Source: CAD feature listing. Evaluate the final solid. Frame: model axes, mm. A direction names the side the tool comes from. Give positions to 0.01 mm unless a question says otherwise; leave off trailing zeros. Loops run counter-clockwise (first coordinate to the right, second up) from the corner with the lowest first, then second, coordinate; pieces in that order, holes last. Notation, with made-up numbers: M 75.25,4 L 89.25,4 A33 cw 89.25,43 Z; hole C 57,5.25 d11. An arc over 180 degrees is marked long. Write item = value, one per line.
from build123d import *

# Parameters (mm, degrees)
BOSS_EXTRUDE1_DEPTH = 38.1
SKETCH2_R           = 19.05
BOSS_EXTRUDE2_DEPTH = 203.2
SKETCH4_W           = 254
SKETCH4_H           = 38.1
BOSS_EXTRUDE3_DEPTH = 177.8
CUT_EXTRUDE3_DEPTH  = 38.1
SKETCH8_R           = 6.35
CUT_EXTRUDE4_DEPTH  = 432.286091243
BOSS_EXTRUDE4_REACH = 409.638
SKETCH9_W           = 50.8
SKETCH9_H           = 38.1
BOSS_EXTRUDE5_DEPTH = 50.8
SKETCH13_W          = 63.5
SKETCH13_H          = 38.1
BOSS_EXTRUDE6_DEPTH = 50.8
CUT_EXTRUDE7_DEPTH  = 438.78172929
FILLET1_R           = 2.54
SKETCH12_R          = 9.525
CUT_EXTRUDE5_DEPTH  = 438.78172929


with BuildPart() as part:
    # Sketch1 → Boss-Extrude1 (new body)
    with BuildSketch(Plane.XY):
        with BuildLine():
            Line((228.6, 38.1), (-228.6, 38.1))
            ThreePointArc((-228.6, 38.1), (-247.65, 19.05), (-228.6, 0))
            Line((-228.6, 0), (228.6, 0))
            ThreePointArc((228.6, 0), (247.65, 19.05), (228.6, 38.1))
        make_face()
    boss_extrude1 = extrude(amount=BOSS_EXTRUDE1_DEPTH)

    # Sketch2 → Boss-Extrude2 (add)
    with BuildSketch(Plane.XY.offset(38.1)):
        with Locations(Location((-228.6, 19.05, 0), (0, 0, 270))):
            Circle(SKETCH2_R)
        with Locations(Location((228.6, 19.05, 0), (0, 0, 90))):
            Circle(SKETCH2_R)
    boss_extrude2 = extrude(amount=BOSS_EXTRUDE2_DEPTH)

    # Mirror3: Boss-Extrude1, Boss-Extrude2 across plane
    add(boss_extrude1.mirror(Plane.XY.offset(139.7)))
    add(boss_extrude2.mirror(Plane.XY.offset(139.7)))

    # Sketch4 → Boss-Extrude3 (add)
    with BuildSketch(Plane(origin=(0, 38.1, 0), x_dir=(1, 0, 0), z_dir=(0, 1, 0))):
        with Locations((-101.6, -260.35)):
            Rectangle(SKETCH4_W, SKETCH4_H)
    boss_extrude3 = extrude(amount=BOSS_EXTRUDE3_DEPTH)

    # Sketch7 → Cut-Extrude3 (cut)
    with BuildSketch(Plane.XY.offset(279.4)):
        Polygon((-228.6, 38.1), (-127, 215.9), (-228.6, 215.9), align=None)
        Polygon((-76.2, 215.9), (25.4, 38.1), (25.4, 215.9), align=None)
        Polygon((-127, 164.704663298), (-199.345521885, 38.1), (-127, 38.1), align=None)
        Polygon((-76.2, 164.704663298), (-76.2, 38.1), (-3.854478115, 38.1), align=None)
    cut_extrude3 = extrude(amount=-CUT_EXTRUDE3_DEPTH, mode=Mode.SUBTRACT)

    # Mirror4: Boss-Extrude3, Cut-Extrude3 across plane
    add(boss_extrude3.mirror(Plane.XY.offset(139.7)))
    add(cut_extrude3.mirror(Plane.XY.offset(139.7)), mode=Mode.SUBTRACT)

    # Sketch8 → Cut-Extrude4 (cut, through all)
    with BuildSketch(Plane.XY.offset(279.4)):
        with Locations((-228.6, 19.05)):
            Circle(SKETCH8_R)
        with Locations((127, 19.05)):
            Circle(SKETCH8_R)
    extrude(amount=-CUT_EXTRUDE4_DEPTH, mode=Mode.SUBTRACT)

    # Sketch9 → Boss-Extrude4 (add, up to next)
    with BuildSketch(Plane(origin=(0, 0, 241.3), x_dir=(-1, 0, 0), z_dir=(0, 0, -1)), mode=Mode.PRIVATE) as boss_extrude4_sk1:
        with Locations((101.6, 196.85)):
            Rectangle(SKETCH9_W, SKETCH9_H)
    boss_extrude4_tool1 = extrude(boss_extrude4_sk1.sketch, amount=BOSS_EXTRUDE4_REACH, mode=Mode.PRIVATE) - part.part
    add(boss_extrude4_tool1.solids().sort_by_distance((-101.6, 196.85, 241.3))[0])

    # Sketch10 → Boss-Extrude5 (add)
    with BuildSketch(Plane.XZ.offset(-177.8)):
        with BuildLine():
            Line((-76.2, 177.8), (-38.1, 177.8))
            Line((-38.1, 177.8), (-38.1, 164.293444248))
            ThreePointArc((-38.1, 164.293444248), (-57.15, 139.7), (-38.1, 115.106555752))
            Line((-38.1, 115.106555752), (-38.1, 101.6))
            Line((-38.1, 101.6), (-76.2, 101.6))
            Line((-76.2, 101.6), (-76.2, 177.8))
        make_face()
    extrude(amount=-BOSS_EXTRUDE5_DEPTH)

    # Sketch13 → Boss-Extrude6 (add)
    with BuildSketch(Plane(origin=(0, 38.1, 0), x_dir=(1, 0, 0), z_dir=(0, 1, 0))):
        with Locations((196.85, -260.35)):
            Rectangle(SKETCH13_W, SKETCH13_H)
        with Locations((196.85, -19.05)):
            Rectangle(SKETCH13_W, SKETCH13_H)
    extrude(amount=BOSS_EXTRUDE6_DEPTH)

    # Sketch14 → Cut-Extrude7 (cut, through all)
    with BuildSketch(Plane(origin=(0, 0, 0), x_dir=(-1, 0, 0), z_dir=(0, 0, -1))):
        Polygon((-177.8, 88.9), (-165.1, 38.1), (-165.1, 88.9), align=None)
        Polygon((-228.6, 38.1), (-215.9, 88.9), (-228.6, 88.9), align=None)
    extrude(amount=-CUT_EXTRUDE7_DEPTH, mode=Mode.SUBTRACT)

    # Fillet1
    # the kernel refuses this fillet: 2.54 mm, written as the material it adds along each edge
    with BuildSketch(Plane(origin=(25.4, 38.1, 38.1), x_dir=(1, 0, 0), z_dir=(0, 0, -1))) as fillet1_piece_1:
        with BuildLine():
            CenterArc((FILLET1_R * 0.580322535471, -FILLET1_R), FILLET1_R, 90, 60.255118703)
            Line((-FILLET1_R * 0.287920606653, -FILLET1_R * 0.503861061643), (0, 0))
            Line((0, 0), (FILLET1_R * 0.580322535471, 0))
        make_face()
    extrude(amount=38.1)
    with BuildSketch(Plane(origin=(-76.2, 215.9, 177.8), x_dir=(-1, 0, 0), z_dir=(0, 0, -1))) as fillet1_piece_2:
        with BuildLine():
            CenterArc((FILLET1_R, FILLET1_R), FILLET1_R, 180, 90)
            Line((0, FILLET1_R), (0, 0))
            Line((0, 0), (FILLET1_R, 0))
        make_face()
    extrude(amount=76.2)
    with BuildSketch(Plane(origin=(165.1, 38.1, 241.3), x_dir=(-1, 0, 0), z_dir=(0, 0, 1))) as fillet1_piece_3:
        with BuildLine():
            CenterArc((FILLET1_R * 0.780776406404, -FILLET1_R), FILLET1_R, 90, 75.963756532)
            Line((-FILLET1_R * 0.189366093741, -FILLET1_R * 0.757464374964), (0, 0))
            Line((0, 0), (FILLET1_R * 0.780776406404, 0))
        make_face()
    extrude(amount=38.1)
    with BuildSketch(Plane(origin=(165.1, 38.1, 38.1), x_dir=(-1, 0, 0), z_dir=(0, 0, -1))) as fillet1_piece_4:
        with BuildLine():
            CenterArc((FILLET1_R * 0.780776406404, FILLET1_R), FILLET1_R, 194.036243468, 75.963756532)
            Line((-FILLET1_R * 0.189366093741, FILLET1_R * 0.757464374964), (0, 0))
            Line((0, 0), (FILLET1_R * 0.780776406404, 0))
        make_face()
    extrude(amount=38.1)
    with BuildSketch(Plane(origin=(-228.6, 38.1, 279.4), x_dir=(-0.9993924886813553, -0.03485188039815198, 0), z_dir=(0, 0, -1))) as fillet1_piece_5:
        with BuildLine():
            CenterArc((1.416380419, 2.538456921), FILLET1_R, 211.742151423, 56.260578451)
            Line((-0.743697302, 1.202169438), (0, 0))
            ThreePointArc((0, 0), (0.663928322, 0.011573091), (1.327856643, 0))
        make_face()
    extrude(amount=38.1)
    with BuildSketch(Plane(origin=(228.6, 38.1, 279.4), x_dir=(0.9989173866825803, -0.04651940007399378, 0), z_dir=(0, 0, -1))) as fillet1_piece_6:
        with BuildLine():
            CenterArc((1.890548419, -2.537250162), FILLET1_R, 92.66632756, 70.631101413)
            Line((-0.542287963, -1.807245273), (0, 0))
            ThreePointArc((0, 0), (0.886194571, -0.020623784), (1.772389143, 0))
        make_face()
    extrude(amount=38.1)
    with BuildSketch(Plane(origin=(25.4, 38.1, 241.3), x_dir=(1, 0, 0), z_dir=(0, 0, 1))) as fillet1_piece_7:
        with BuildLine():
            CenterArc((FILLET1_R * 0.580322535471, FILLET1_R), FILLET1_R, 209.744881297, 60.255118703)
            Line((-FILLET1_R * 0.287920606653, FILLET1_R * 0.503861061643), (0, 0))
            Line((0, 0), (FILLET1_R * 0.580322535471, 0))
        make_face()
    extrude(amount=38.1)
    with BuildSketch(Plane(origin=(-228.6, 38.1, 0), x_dir=(-0.9993924886813553, -0.03485188039815198, 0), z_dir=(0, 0, 1))) as fillet1_piece_8:
        with BuildLine():
            CenterArc((1.416380419, -2.538456921), FILLET1_R, 91.997270126, 56.260578451)
            Line((-0.743697302, -1.202169438), (0, 0))
            ThreePointArc((0, 0), (0.663928322, -0.011573091), (1.327856643, 0))
        make_face()
    extrude(amount=38.1)
    with BuildSketch(Plane(origin=(228.6, 38.1, 0), x_dir=(0.9989173866825803, -0.04651940007399378, 0), z_dir=(0, 0, 1))) as fillet1_piece_9:
        with BuildLine():
            CenterArc((1.890548419, 2.537250162), FILLET1_R, 196.702571028, 70.631101413)
            Line((-0.542287963, 1.807245273), (0, 0))
            ThreePointArc((0, 0), (0.886194571, 0.020623784), (1.772389143, 0))
        make_face()
    extrude(amount=38.1)
    # the kernel refuses this fillet: 2.54 mm, written as the material it takes off along each edge
    with BuildSketch(Plane(origin=(215.9, 88.9, -4.957930181), x_dir=(0.2425356250363313, -0.9701425001453323, 0), z_dir=(0, 0, 1)), Plane(origin=(177.8, 88.9, -4.957930181), x_dir=(1, 0, 0), z_dir=(0, 0, 1))) as fillet1_2_piece_1:
        with BuildLine():
            CenterArc((FILLET1_R * 0.780776406404, -FILLET1_R), FILLET1_R, 90, 75.963756532)
            Line((-FILLET1_R * 0.189366093741, -FILLET1_R * 0.757464374964), (0, 0))
            Line((0, 0), (FILLET1_R * 0.780776406404, 0))
        make_face()
    extrude(amount=48.015860361, mode=Mode.SUBTRACT)
    with BuildSketch(Plane(origin=(177.8, 88.9, 236.342069819), x_dir=(-0.2425356250363296, -0.9701425001453328, 0), z_dir=(0, 0, 1)), Plane(origin=(215.9, 88.9, 236.342069819), x_dir=(-1, 0, 0), z_dir=(0, 0, 1))) as fillet1_2_piece_2:
        with BuildLine():
            CenterArc((FILLET1_R * 0.780776406404, FILLET1_R), FILLET1_R, 194.036243468, 75.963756532)
            Line((-FILLET1_R * 0.189366093741, FILLET1_R * 0.757464374964), (0, 0))
            Line((0, 0), (FILLET1_R * 0.780776406404, 0))
        make_face()
    extrude(amount=48.015860361, mode=Mode.SUBTRACT)

    # Sketch12 → Cut-Extrude5 (cut, through all)
    with BuildSketch(Plane(origin=(0, 0, 0), x_dir=(-1, 0, 0), z_dir=(0, 0, -1))):
        with Locations((41.275, 18.386071678)):
            Circle(SKETCH12_R)
        with Locations((-196.85, 63.5)):
            Circle(SKETCH12_R)
    extrude(amount=-CUT_EXTRUDE5_DEPTH, mode=Mode.SUBTRACT)


solid = part.part
1. Cut plane C-C, the plane x = 196.85. Return the cut outline in (y, z) (3 decimals).
Derived:
outline = M 0,0 L 53.975,0 L 53.975,38.1 L 0,38.1 Z; M 0,241.3 L 53.975,241.3 L 53.975,279.4 L 0,279.4 Z; M 73.025,0 L 88.9,0 L 88.9,38.1 L 73.025,38.1 Z; M 73.025,241.3 L 88.9,241.3 L 88.9,279.4 L 73.025,279.4 Z
2. First-contact query: pin 1 Ø1 at (x, z) = (-103, 163.5) entering from +Y; pin 2 Ø11.5 at (y, z) = (72, 15.5) entering from -X; pin 3 Ø11.5 at (x, y) = (-41.28, 18.39) entering from +Z; pin 4 Ø7 at (y, z) = (205.5, 108) entering from +X. Flat tips, straight axial feed; report the tip coordinate or a pass-through.
Derived:
pin_1 = 215.9
pin_2 = -212.51
pin_3 = through
pin_4 = -38.1
3. Cut plane D-D, the plane z = 152.5. Return the cut outline in (x, y), then the cut area to 3 significant figures.
Derived:
outline = C -228.6,19.05 d38.1; M -127,177.8 L -53.69,177.8 L -53.69,228.6 L -76.2,228.6 L -76.2,218.44 A2.54 cw -78.74,215.9 L -127,215.9 Z; C 228.6,19.05 d38.1; hole C -228.6,19.05 d12.7
area = 5,230 mm²
4. Pull-direction query (Y, two-part tool) for faces 1 (the flat face through (-39.521, 100.516, 260.617)), 2 (the flat face through (-3, 0, 261)), 3 (the flat face through (3, 61, 241.3)); classes: +Y half, -Y half, draft (parallel to the pull), parting line (faces both ways), or undercut.
Derived:
face_1 = undercut
face_2 = -Y half
face_3 = draft
5. Cut plane B-B, the plane x = 54.5. Return the cut outline in (y, z), then the cut area to 3 significant figures.
Derived:
outline = M 0,0 L 38.1,0 L 38.1,38.1 L 0,38.1 Z; M 0,241.3 L 38.1,241.3 L 38.1,279.4 L 0,279.4 Z
area = 2,900 mm²
6. Material intervals for probe 1 along Z at (x, y) = (-124.5, 123); probe 2 along Y at (x, z) = (196, 252); probe 3 along X at (y, z) = (17, 245.5), sorted ascending. Write a range as from..to.
Derived:
probe_1 = 0..38.1, 241.3..279.4
probe_2 = 0..54.01, 72.99..88.9
probe_3 = -247.54..-234.61, -222.59..-50.7, -31.85..120.99, 133.01..247.54
7. Cut plane A-A, the plane z = 215.5. Return the cut outline in (x, y).
Derived:
outline = C -228.6,19.05 d38.1; M -127,177.8 L -76.2,177.8 L -76.2,215.9 L -127,215.9 Z; C 228.6,19.05 d38.1; hole C -228.6,19.05 d12.7
8. Reachability of faces 4 (the flat face through (-26.472, 128.876, 18.783)), 5 (the flat face through (-76.2, 102, 19)), 6 (the flat face through (171.532, 63.829, 260.083)) from +Z, -Z, +X, -X, +Y, -Y: full face, straight path, thin tool, end or side. Return the list, or none.
Derived:
face_4 = -Z, +Y
face_5 = +Z, -Z
face_6 = +Z, -Z, +Y
